```python
from build123d import *

# Parameters (mm, degrees)
SKETCH1_W           = 50.8
SKETCH1_H           = 101.6
SKETCH1_R           = 1.0795
BOSS_EXTRUDE1_DEPTH = 3.175
SKETCH3_R           = 0.79375
CUT_EXTRUDE1_DEPTH  = 6.35
SKETCH4_R           = 0.79375
CUT_EXTRUDE2_DEPTH  = 3.81
SKETCH5_R           = 3.175
CUT_EXTRUDE3_DEPTH  = 4.175
SKETCH6_R           = 1.4605
CUT_EXTRUDE4_DEPTH  = 4.175


with BuildPart() as part:
    # Sketch1 → Boss-Extrude1 (new body)
    with BuildSketch(Plane.XY):
        with Locations((-30.443913465, -14.686809816)):
            Rectangle(SKETCH1_W, SKETCH1_H)
        with Locations((-53.113413465, 33.382690184)):
            Circle(SKETCH1_R, mode=Mode.SUBTRACT)
        with Locations((-53.113413465, -62.756309816)):
            Circle(SKETCH1_R, mode=Mode.SUBTRACT)
        with Locations((-7.774413465, -62.756309816)):
            Circle(SKETCH1_R, mode=Mode.SUBTRACT)
        with Locations((-7.774413465, 33.382690184)):
            Circle(SKETCH1_R, mode=Mode.SUBTRACT)
    extrude(amount=BOSS_EXTRUDE1_DEPTH)

    # Sketch3 → Cut-Extrude1 (cut)
    with BuildSketch(Plane(origin=(0, 36.113190184, 0), x_dir=(1, 0, 0), z_dir=(0, 1, 0))):
        with Locations(Location((-30.443913465, -1.5875, 0), (0, 0, 270))):  # turned: the seam where the file's is
            Circle(SKETCH3_R)
    extrude(amount=-CUT_EXTRUDE1_DEPTH, mode=Mode.SUBTRACT)

    # Sketch4 → Cut-Extrude2 (cut)
    with BuildSketch(Plane(origin=(0, -65.486809816, 0), x_dir=(-1, 0, 0), z_dir=(0, -1, 0))):
        with Locations(Location((30.443913465, -1.5875, 0), (0, 0, 270))):  # turned: the seam where the file's is
            Circle(SKETCH4_R)
    extrude(amount=-CUT_EXTRUDE2_DEPTH, mode=Mode.SUBTRACT)

    # Sketch5 → Cut-Extrude3 (cut, through all)
    with BuildSketch(Plane.XY.offset(3.175)):
        with Locations((-30.443913465, -1.986809816)):
            Circle(SKETCH5_R)
    extrude(amount=-CUT_EXTRUDE3_DEPTH, mode=Mode.SUBTRACT)

    # Sketch6 → Cut-Extrude4 (cut, through all)
    with BuildSketch(Plane.XY.offset(3.175)):
        with Locations((-39.143413465, -40.086809816)):
            Circle(SKETCH6_R)
        with Locations((-21.744413465, -40.086809816)):
            Circle(SKETCH6_R)
    extrude(amount=-CUT_EXTRUDE4_DEPTH, mode=Mode.SUBTRACT)


solid = part.part
```
Input: part model. Units: mm. Frame: model coordinates. Give positions to 0.01 mm unless a question says otherwise; leave off trailing zeros. Order: outer loops, then holes, each group sorted by start corner. A loop starts at its lowest first (then second) coordinate and runs counter-clockwise, first axis right, second up.
1. Pin query (flat end, axial travel): pin 1 (1.7 mm diameter, centred on x = -53.11, y = -62.76, fed in from -Z) (3 decimals); pin 2 (0.5 mm diameter, centred on x = -30, z = 1.5, fed in from -Y); pin 3 (6 mm diameter, centred on x = -42.5, y = 22.5, fed in from -Z); pin 4 (0.5 mm diameter, centred on x = -30.5, z = 1.5, fed in from +Y). Return the tip coordinate at first contact, or that it passes through.
Derived:
pin 1: passes through
pin 2: stops at y = -61.68
pin 3: stops at z = 0
pin 4: stops at y = 29.76
2. Material intervals for L1, parallel to Y at x = -32, z = 2.65; L2, parallel to Y at x = -30, z = 1.95, sorted ascending.
Derived:
L1: y = -65.49 to -4.75, 0.78 to 36.11
L2: y = -61.68 to -5.13, 1.16 to 29.76
3. Section A-A on y = -4. Return the cut outline in (x, z) (3 decimals), and give its area (3 significant figures).
Derived:
outline: (-55.844, 0) - (-32.899, 0) - (-32.899, 3.175) - (-55.844, 3.175) - close; (-27.989, 0) - (-5.044, 0) - (-5.044, 3.175) - (-27.989, 3.175) - close
area: 146 mm2
